Part model, mm, in its own coordinate system. Round coordinates to 2 decimals unless told otherwise and drop trailing zeros. Write each loop counter-clockwise with the first axis right and the second up, starting at its lowest first coordinate (ties: lowest second). Pieces come first, ordered by that corner, then holes. Notation, with made-up numbers: (82, 74.5) -> (111, 74.5) arc R23 cw to (111, 109.5) -> close; hole circle Ø6 at (8, 55.25). An arc over 180 degrees is marked (long way). Return JSON: item names as keys, results as strings. Group by question number.
```python
from build123d import *

# Parameters (mm, degrees)
SKETCH1_W               = 137.16
SKETCH1_H               = 114.3
BOSS_EXTRUDE1_DEPTH     = 1.5875
SKETCH2_R               = 2.794
CUT_EXTRUDE2_DEPTH      = 90.285267857
CAVITY7_START           = -68.58
CAVITY7_OUTLINE_W       = 4.9609375
CAVITY7_OUTLINE_H       = 1.5875
CAVITY7_DEPTH           = 15.24
CAVITY7_START_2         = -38.1
CAVITY7_2_OUTLINE_W     = 4.9609375
CAVITY7_2_OUTLINE_H     = 1.5875
CAVITY7_2_DEPTH         = 15.24
CAVITY7_START_3         = -7.62
CAVITY7_3_OUTLINE_W     = 4.9609375
CAVITY7_3_OUTLINE_H     = 1.5875
CAVITY7_3_DEPTH         = 15.24
CAVITY7_START_4         = 22.86
CAVITY7_4_OUTLINE_W     = 4.9609375
CAVITY7_4_OUTLINE_H     = 1.5875
CAVITY7_4_DEPTH         = 15.24
CAVITY7_START_5         = 53.34
CAVITY7_5_OUTLINE_W     = 4.9609375
CAVITY7_5_OUTLINE_H     = 1.5875
CAVITY7_5_DEPTH         = 15.24
CAVITY8_START           = -68.58
CAVITY8_OUTLINE_W       = 4.9609375
CAVITY8_OUTLINE_H       = 1.5875
CAVITY8_DEPTH           = 15.24
CAVITY8_START_2         = -38.1
CAVITY8_2_OUTLINE_W     = 4.9609375
CAVITY8_2_OUTLINE_H     = 1.5875
CAVITY8_2_DEPTH         = 15.24
CAVITY8_START_3         = -7.62
CAVITY8_3_OUTLINE_W     = 4.9609375
CAVITY8_3_OUTLINE_H     = 1.5875
CAVITY8_3_DEPTH         = 15.24
CAVITY8_START_4         = 22.86
CAVITY8_4_OUTLINE_W     = 4.9609375
CAVITY8_4_OUTLINE_H     = 1.5875
CAVITY8_4_DEPTH         = 15.24
CAVITY8_START_5         = 53.34
CAVITY8_5_OUTLINE_W     = 4.9609375
CAVITY8_5_OUTLINE_H     = 1.5875
CAVITY8_5_DEPTH         = 15.24
CAVITY9_START           = -68.58
CAVITY9_OUTLINE_W       = 7.7390625
CAVITY9_OUTLINE_H       = 1.5875
CAVITY9_OUTLINE_W_2     = 12.7
CAVITY9_DEPTH           = 4.9609375
CAVITY10_START          = -31.75
CAVITY10_OUTLINE_W      = 4.9609375
CAVITY10_OUTLINE_H      = 1.5875
CAVITY10_DEPTH          = 12.7
CAVITY10_START_2        = -6.35
CAVITY10_2_OUTLINE_W    = 4.9609375
CAVITY10_2_OUTLINE_H    = 1.5875
CAVITY10_2_DEPTH        = 12.7
CAVITY10_START_3        = 19.05
CAVITY10_3_OUTLINE_W    = 4.9609375
CAVITY10_3_OUTLINE_H    = 1.5875
CAVITY10_3_DEPTH        = 12.7
CAVITY10_START_4        = -52.1890625
CAVITY10_4_OUTLINE_W    = 4.9609375
CAVITY10_4_OUTLINE_H    = 1.5875
CAVITY10_4_DEPTH        = 7.7390625
CAVITY10_START_5        = 44.45
CAVITY10_5_OUTLINE_W    = 4.9609375
CAVITY10_5_OUTLINE_H    = 1.5875
CAVITY10_5_DEPTH        = 7.7390625
CUT_EXTRUDE6_DEPTH      = 90.285267857
CUT_EXTRUDE6_DEPTH_BACK = 90.285267857
SKETCH3_W               = 10.1854
SKETCH3_H               = 2.5908
SKETCH5_R               = 1.0922
CUT_EXTRUDE7_DEPTH      = 90.285267857
SKETCH6_R               = 1.0922
CUT_EXTRUDE8_DEPTH      = 90.285267857
SKETCH7_R               = 1.0922
CUT_EXTRUDE9_DEPTH      = 90.285267857
SKETCH8_R               = 1.0922
CUT_EXTRUDE10_DEPTH     = 90.285267857
SKETCH9_R               = 1.0922
CUT_EXTRUDE11_DEPTH     = 90.285267857
SKETCH10_R              = 1.0922
CUT_EXTRUDE12_DEPTH     = 90.285267857


# Read off the part's stored shape, not the designer's step: Cavity7, Cavity8, Cavity9, Cavity10
with BuildPart() as part:
    # Sketch1 → Boss-Extrude1 (new body)
    with BuildSketch(Plane.XY):
        Rectangle(SKETCH1_W, SKETCH1_H)
    extrude(amount=BOSS_EXTRUDE1_DEPTH)

    # Sketch2 → Cut-Extrude2 (cut, through all)
    with BuildSketch(Plane.XY.offset(1.5875)):
        with Locations((0, 40.64)):
            Circle(SKETCH2_R)
    extrude(amount=-CUT_EXTRUDE2_DEPTH, mode=Mode.SUBTRACT)

    # Cavity7 outline → Cavity7 (cut)
    with BuildSketch(Plane.YZ.offset(CAVITY7_START)):
        with Locations((-54.66953125, 0.79375)):
            Rectangle(CAVITY7_OUTLINE_W, CAVITY7_OUTLINE_H)
    extrude(amount=CAVITY7_DEPTH, mode=Mode.SUBTRACT)

    # Cavity7 2 outline → Cavity7 2 (cut)
    with BuildSketch(Plane.YZ.offset(CAVITY7_START_2)):
        with Locations((-54.66953125, 0.79375)):
            Rectangle(CAVITY7_2_OUTLINE_W, CAVITY7_2_OUTLINE_H)
    extrude(amount=CAVITY7_2_DEPTH, mode=Mode.SUBTRACT)

    # Cavity7 3 outline → Cavity7 3 (cut)
    with BuildSketch(Plane.YZ.offset(CAVITY7_START_3)):
        with Locations((-54.66953125, 0.79375)):
            Rectangle(CAVITY7_3_OUTLINE_W, CAVITY7_3_OUTLINE_H)
    extrude(amount=CAVITY7_3_DEPTH, mode=Mode.SUBTRACT)

    # Cavity7 4 outline → Cavity7 4 (cut)
    with BuildSketch(Plane.YZ.offset(CAVITY7_START_4)):
        with Locations((-54.66953125, 0.79375)):
            Rectangle(CAVITY7_4_OUTLINE_W, CAVITY7_4_OUTLINE_H)
    extrude(amount=CAVITY7_4_DEPTH, mode=Mode.SUBTRACT)

    # Cavity7 5 outline → Cavity7 5 (cut)
    with BuildSketch(Plane.YZ.offset(CAVITY7_START_5)):
        with Locations((-54.66953125, 0.79375)):
            Rectangle(CAVITY7_5_OUTLINE_W, CAVITY7_5_OUTLINE_H)
    extrude(amount=CAVITY7_5_DEPTH, mode=Mode.SUBTRACT)

    # Cavity8 outline → Cavity8 (cut)
    with BuildSketch(Plane.YZ.offset(CAVITY8_START)):
        with Locations((54.66953125, 0.79375)):
            Rectangle(CAVITY8_OUTLINE_W, CAVITY8_OUTLINE_H)
    extrude(amount=CAVITY8_DEPTH, mode=Mode.SUBTRACT)

    # Cavity8 2 outline → Cavity8 2 (cut)
    with BuildSketch(Plane.YZ.offset(CAVITY8_START_2)):
        with Locations((54.66953125, 0.79375)):
            Rectangle(CAVITY8_2_OUTLINE_W, CAVITY8_2_OUTLINE_H)
    extrude(amount=CAVITY8_2_DEPTH, mode=Mode.SUBTRACT)

    # Cavity8 3 outline → Cavity8 3 (cut)
    with BuildSketch(Plane.YZ.offset(CAVITY8_START_3)):
        with Locations((54.66953125, 0.79375)):
            Rectangle(CAVITY8_3_OUTLINE_W, CAVITY8_3_OUTLINE_H)
    extrude(amount=CAVITY8_3_DEPTH, mode=Mode.SUBTRACT)

    # Cavity8 4 outline → Cavity8 4 (cut)
    with BuildSketch(Plane.YZ.offset(CAVITY8_START_4)):
        with Locations((54.66953125, 0.79375)):
            Rectangle(CAVITY8_4_OUTLINE_W, CAVITY8_4_OUTLINE_H)
    extrude(amount=CAVITY8_4_DEPTH, mode=Mode.SUBTRACT)

    # Cavity8 5 outline → Cavity8 5 (cut)
    with BuildSketch(Plane.YZ.offset(CAVITY8_START_5)):
        with Locations((54.66953125, 0.79375)):
            Rectangle(CAVITY8_5_OUTLINE_W, CAVITY8_5_OUTLINE_H)
    extrude(amount=CAVITY8_5_DEPTH, mode=Mode.SUBTRACT)

    # Cavity9 outline → Cavity9 (cut)
    with BuildSketch(Plane.YZ.offset(CAVITY9_START)):
        with Locations((48.31953125, 0.79375)):
            Rectangle(CAVITY9_OUTLINE_W, CAVITY9_OUTLINE_H)
        with Locations((25.4, 0.79375)):
            Rectangle(CAVITY9_OUTLINE_W_2, CAVITY9_OUTLINE_H)
        with Locations((0, 0.79375)):
            Rectangle(CAVITY9_OUTLINE_W_2, CAVITY9_OUTLINE_H)
        with Locations((-25.4, 0.79375)):
            Rectangle(CAVITY9_OUTLINE_W_2, CAVITY9_OUTLINE_H)
        with Locations((-48.31953125, 0.79375)):
            Rectangle(CAVITY9_OUTLINE_W, CAVITY9_OUTLINE_H)
    extrude(amount=CAVITY9_DEPTH, mode=Mode.SUBTRACT)

    # Cavity10 outline → Cavity10 (cut)
    with BuildSketch(Plane(origin=(0, 0, 0), x_dir=(1, 0, 0), z_dir=(0, 1, 0)).offset(CAVITY10_START)):
        with Locations((66.09953125, -0.79375)):
            Rectangle(CAVITY10_OUTLINE_W, CAVITY10_OUTLINE_H)
    extrude(amount=CAVITY10_DEPTH, mode=Mode.SUBTRACT)

    # Cavity10 2 outline → Cavity10 2 (cut)
    with BuildSketch(Plane(origin=(0, 0, 0), x_dir=(1, 0, 0), z_dir=(0, 1, 0)).offset(CAVITY10_START_2)):
        with Locations((66.09953125, -0.79375)):
            Rectangle(CAVITY10_2_OUTLINE_W, CAVITY10_2_OUTLINE_H)
    extrude(amount=CAVITY10_2_DEPTH, mode=Mode.SUBTRACT)

    # Cavity10 3 outline → Cavity10 3 (cut)
    with BuildSketch(Plane(origin=(0, 0, 0), x_dir=(1, 0, 0), z_dir=(0, 1, 0)).offset(CAVITY10_START_3)):
        with Locations((66.09953125, -0.79375)):
            Rectangle(CAVITY10_3_OUTLINE_W, CAVITY10_3_OUTLINE_H)
    extrude(amount=CAVITY10_3_DEPTH, mode=Mode.SUBTRACT)

    # Cavity10 4 outline → Cavity10 4 (cut)
    with BuildSketch(Plane(origin=(0, 0, 0), x_dir=(1, 0, 0), z_dir=(0, 1, 0)).offset(CAVITY10_START_4)):
        with Locations((66.09953125, -0.79375)):
            Rectangle(CAVITY10_4_OUTLINE_W, CAVITY10_4_OUTLINE_H)
    extrude(amount=CAVITY10_4_DEPTH, mode=Mode.SUBTRACT)

    # Cavity10 5 outline → Cavity10 5 (cut)
    with BuildSketch(Plane(origin=(0, 0, 0), x_dir=(1, 0, 0), z_dir=(0, 1, 0)).offset(CAVITY10_START_5)):
        with Locations((66.09953125, -0.79375)):
            Rectangle(CAVITY10_5_OUTLINE_W, CAVITY10_5_OUTLINE_H)
    extrude(amount=CAVITY10_5_DEPTH, mode=Mode.SUBTRACT)

    # Sketch3 → Cut-Extrude6 (cut, two sides: drawn at the far end of the back side and taken through both)
    with BuildSketch(Plane.XY.offset(1.5875).offset(-CUT_EXTRUDE6_DEPTH_BACK)):
        with Locations((0.061, -20.75)):
            Rectangle(SKETCH3_W, SKETCH3_H)
    extrude(amount=CUT_EXTRUDE6_DEPTH + CUT_EXTRUDE6_DEPTH_BACK, mode=Mode.SUBTRACT)

    # Sketch5 → Cut-Extrude7 (cut, through all)
    with BuildSketch(Plane.XY.offset(1.5875)):
        with Locations((-10.289, -21.1)):
            Circle(SKETCH5_R)
    extrude(amount=-CUT_EXTRUDE7_DEPTH, mode=Mode.SUBTRACT)

    # Sketch6 → Cut-Extrude8 (cut, through all)
    with BuildSketch(Plane.XY.offset(1.5875)):
        with Locations((10.411, -21.1)):
            Circle(SKETCH6_R)
    extrude(amount=-CUT_EXTRUDE8_DEPTH, mode=Mode.SUBTRACT)

    # Sketch7 → Cut-Extrude9 (cut, through all)
    with BuildSketch(Plane.XY.offset(1.5875)):
        with Locations((10.411, -44.3)):
            Circle(SKETCH7_R)
    extrude(amount=-CUT_EXTRUDE9_DEPTH, mode=Mode.SUBTRACT)

    # Sketch8 → Cut-Extrude10 (cut, through all)
    with BuildSketch(Plane.XY.offset(1.5875)):
        with Locations((-10.289, -44.3)):
            Circle(SKETCH8_R)
    extrude(amount=-CUT_EXTRUDE10_DEPTH, mode=Mode.SUBTRACT)

    # Sketch9 → Cut-Extrude11 (cut, through all)
    with BuildSketch(Plane.XY.offset(1.5875)):
        with Locations((60.5710625, 49.1410625)):
            Circle(SKETCH9_R)
        with Locations((13.8350625, 49.1410625)):
            Circle(SKETCH9_R)
        with Locations((13.8350625, -17.5339375)):
            Circle(SKETCH9_R)
        with Locations((60.5710625, -17.5339375)):
            Circle(SKETCH9_R)
        with Locations((-13.4286625, 49.1410625)):
            Circle(SKETCH9_R)
        with Locations((-60.5710625, 49.1410625)):
            Circle(SKETCH9_R)
        with Locations((-60.5710625, -17.5339375)):
            Circle(SKETCH9_R)
        with Locations((-13.4286625, -17.5339375)):
            Circle(SKETCH9_R)
    extrude(amount=-CUT_EXTRUDE11_DEPTH, mode=Mode.SUBTRACT)

    # Sketch10 → Cut-Extrude12 (cut, through all)
    with BuildSketch(Plane.XY.offset(1.5875)):
        with Locations((-6.214337236, 46.854337236)):
            Circle(SKETCH10_R)
        with Locations((6.214337236, 46.854337236)):
            Circle(SKETCH10_R)
    extrude(amount=-CUT_EXTRUDE12_DEPTH, mode=Mode.SUBTRACT)


solid = part.part
```
Item 1: Cut at D-D (z = 0.4). State how many separate pieces and enclosed holes the cut face has, then the cut area to 3 significant figures.
Item 2: Two-plate mould, pull along X, no slides. Class faces 1 (the face through (-1, 1, 0)), 2 (the face through (-0.606, 37.912, 0.805)): released by +X, released by -X, zero draft, split by the parting line, or undercut.
Item 3: Cut at A-A (y = 40.64). Write the cut outline in (x, z).
Item 4: Flat gauge pins, fed straight in: P1, Ø0.5, axis at x = -29.5, z = 1, coming from the +Y side; P2, Ø0.5, axis at y = -47, z = 0.5, coming from the -X side; P3, Ø0.5, axis at y = -55, z = 1, coming from the +X side; P4, Ø4.5, axis at x = 0, y = 40.64, coming from the +Z side. Where does each tip first touch, or does it go through?
Item 5: Wall check: L1, parallel to X at y = 52.5, z = 1.25; L2, parallel to X at y = 44.5, z = 1.35; L3, parallel to Y at x = -5, z = 0.65. Give the ranges that are in metal, low to high.
Item 6: Cut at B-B (x = -25). Write the cut outline in (y, z), then the cut area to 3 significant figures.
Item 7: Cut at C-C (y = -30). Write the cut outline in (x, z), then the cut area to 3 significant figures.
Checks:
{
 "1": {"separate pieces": "1", "enclosed holes": "16", "area": "14,300 mm2"},
 "2": {"face 1": "zero draft", "face 2": "undercut"},
 "3": {"outline": "(-68.58, 0) -> (-2.79, 0) -> (-2.79, 1.59) -> (-68.58, 1.59) -> close; (2.79, 0) -> (68.58, 0) -> (68.58, 1.59) -> (2.79, 1.59) -> close"},
 "4": {"P1": "stops at y = 52.19", "P2": "stops at x = -63.62", "P3": "stops at x = 53.34", "P4": "passes through"},
 "5": {"L1": "x = -53.34 to -38.1, -22.86 to -7.62, 7.62 to 22.86, 38.1 to 53.34", "L2": "x = -63.62 to 63.62", "L3": "y = -52.19 to -22.05, -19.45 to 52.19"},
 "6": {"outline": "(-52.19, 0) -> (52.19, 0) -> (52.19, 1.59) -> (-52.19, 1.59) -> close", "area": "166 mm2"},
 "7": {"outline": "(-63.62, 0) -> (63.62, 0) -> (63.62, 1.59) -> (-63.62, 1.59) -> close", "area": "202 mm2"}
}
